Here's how the part is built. I have some questions about the finished solid (model axes, mm). A direction names the side the tool comes from. Coordinates: 2 decimals unless noted, no trailing zeros. Loops run counter-clockwise (first coordinate to the right, second up) from the corner with the lowest first, then second, coordinate; pieces in that order, holes last. Notation, with made-up numbers: (47, 73.25) - (81, 73.25) arc R19 ccw to (81, 88.25) - close; hole circle Ø7 at (-16.75, -38.75). An arc over 180 degrees is marked (long way). Use a Markdown table: item, result.
```python
from build123d import *

# Parameters (mm, degrees)
SKETCH1_W          = 50.8
SKETCH1_H          = 28.575
EXTRUDE1_DEPTH     = 65.8368
LPATTERN1_COUNT    = 2
LPATTERN1_PITCH    = 46.99
SKETCH5_R          = 13.5001
EXTRUDE2_DEPTH     = 5.969
SKETCH6_W          = 6.3373
SKETCH6_H          = 16.891
CUT_EXTRUDE4_DEPTH = 30.48
HOLE1_D            = 7.137
HOLE1_DEPTH        = 65.8368
HOLE2_D            = 7.137
HOLE2_DEPTH        = 28.575
EXTRUDE3_DEPTH     = 6.78


with BuildPart() as part:
    # Sketch1 → Extrude1 (new body)
    with BuildSketch(Plane(origin=(0, 0, 0), x_dir=(0, 0, -1), z_dir=(1, 0, 0))):
        with Locations((2.3876, 0)):
            Rectangle(SKETCH1_W, SKETCH1_H)
    extrude(amount=EXTRUDE1_DEPTH)

    # S2D0002 → Cut-Revolve1 (revolve, cut)
    with BuildSketch(Plane(origin=(0, 4.7625, 0), x_dir=(-1, 0, 0), z_dir=(0, 1, 0)), mode=Mode.PRIVATE) as cut_revolve1_sk:
        Polygon((-14.5415, -27.5336), (-18.161, -27.5336), (-18.161, -27.7876), (-9.525, -27.7876), (-9.525, -14.0716), (-13.9446, -14.0716), (-13.9446, -26.9113), (-14.5415, -27.5082), align=None)
    cut_revolve1 = revolve(cut_revolve1_sk.sketch.rotate(Axis((9.525, 4.7625, -19.13842003), (0, 0, 1)), 180), axis=Axis((9.525, 4.7625, -19.13842003), (0, 0, 1)), mode=Mode.SUBTRACT)  # turned: the seam where the file's is

    # LPattern1: Cut-Revolve1 ×2
    with Locations(*[(i * LPATTERN1_PITCH, 0, 0) for i in range(1, LPATTERN1_COUNT)]):
        add(cut_revolve1, mode=Mode.SUBTRACT)

    # Sketch5 → Extrude2 (add)
    with BuildSketch(Plane.ZY):
        Circle(SKETCH5_R)
    extrude(amount=EXTRUDE2_DEPTH)

    # Sketch6 → Revolve1 (revolve)
    with BuildSketch(Plane(origin=(0, 0, 0), x_dir=(0, 0, 1), z_dir=(0, -1, 0)), mode=Mode.PRIVATE) as revolve1_sk:
        with Locations((-3.16865, 14.4145)):
            Rectangle(SKETCH6_W, SKETCH6_H)
    revolve(revolve1_sk.sketch.rotate(Axis((5.754582971, 0, 0), (-1, 0, 0)), 180), axis=Axis((5.754582971, 0, 0), (-1, 0, 0)))  # turned: the seam where the file's is

    # S2D0001 → Cut-Revolve4 (revolve, cut)
    with BuildSketch(Plane(origin=(-18.511260017, 3.2639, 0), x_dir=(0, 1, 0), z_dir=(0, 0, 1)), mode=Mode.PRIVATE) as cut_revolve4_sk:
        Polygon((-0.7493, 2.984923177), (-0.7493, -11.653260017), (-3.2639, -13.16418413), (-3.2639, 4.348739983), (0.0381, 4.348739983), align=None)
    revolve(cut_revolve4_sk.sketch.rotate(Axis((0, 0, 0), (-1, 0, 0)), 90), axis=Axis((0, 0, 0), (-1, 0, 0)), mode=Mode.SUBTRACT)  # turned: the seam where the file's is

    # Sketch8 → Cut-Revolve5 (revolve, cut)
    with BuildSketch(Plane(origin=(0, 0, 0), x_dir=(0, 0, -1), z_dir=(0, 1, 0)), mode=Mode.PRIVATE) as cut_revolve5_sk:
        with BuildLine():
            Line((-6.3373, 16.5354), (-6.096, 17.2974))
            Line((-6.096, 17.2974), (-6.096, 21.844))
            ThreePointArc((-6.096, 21.844), (-5.995678675, 22.387796865), (-5.707922533, 22.86))
            Line((-5.707922533, 22.86), (-6.3373, 22.86))
            Line((-6.3373, 22.86), (-6.3373, 16.5354))
        make_face()
    revolve(cut_revolve5_sk.sketch.rotate(Axis((-12.65936, 0, 0), (-1, 0, 0)), 180), axis=Axis((-12.65936, 0, 0), (-1, 0, 0)), mode=Mode.SUBTRACT)  # turned: the seam where the file's is

    # Sketch12 → Cut-Extrude4 (cut, symmetric)
    with BuildSketch(Plane(origin=(0, 0, 0), x_dir=(0, -1, 0), z_dir=(0, 0, -1))):
        Polygon((5.461, 22.86), (5.461, 18.0848), (6.096, 17.4498), (6.096, 22.86), align=None)
        Polygon((-5.461, 22.86), (-5.461, 18.0848), (-6.096, 17.4498), (-6.096, 22.86), align=None)
    extrude(amount=CUT_EXTRUDE4_DEPTH, both=True, mode=Mode.SUBTRACT)

    # Hole1
    with Locations(Plane.ZY):
        with Locations((-16.6878, -7.9248), (16.6624, 7.9502)):
            Hole(HOLE1_D / 2, depth=HOLE1_DEPTH)

    # Hole2
    with Locations(Plane(origin=(0, 14.2875, 0), x_dir=(-1, 0, 0), z_dir=(0, 1, 0))):
        with Locations((-23.3172, -16.6878), (-23.3172, 16.6624)):
            Hole(HOLE2_D / 2, depth=HOLE2_DEPTH)

    # Sketch18 → Extrude3 (add)
    with BuildSketch(Plane(origin=(0, 0, -27.5336), x_dir=(-1, 0, 0), z_dir=(0, 0, -1))):
        Polygon((-2.54, 8.79529163), (-9.525, 12.828083261), (-16.51, 8.79529163), (-16.51, 0.72970837), (-9.525, -3.303083261), (-2.54, 0.72970837), align=None)
    extrude(amount=EXTRUDE3_DEPTH)

    # Sketch19 → Cut-Revolve6 (revolve, cut)
    with BuildSketch(Plane(origin=(0, 4.7625, 0), x_dir=(-1, 0, 0), z_dir=(0, 1, 0)), mode=Mode.PRIVATE) as cut_revolve6_sk:
        with BuildLine():
            Line((-15.748, -34.3136), (-15.748, -36.7266))
            Line((-15.748, -36.7266), (-18.923, -36.7266))
            Line((-18.923, -36.7266), (-18.923, -33.5516))
            Line((-18.923, -33.5516), (-16.51, -33.5516))
            ThreePointArc((-16.51, -33.5516), (-16.286815367, -34.090415367), (-15.748, -34.3136))
        make_face()
    revolve(cut_revolve6_sk.sketch.rotate(Axis((9.525, 4.7625, -18.51025594), (0, 0, -1)), 180), axis=Axis((9.525, 4.7625, -18.51025594), (0, 0, -1)), mode=Mode.SUBTRACT)  # turned: the seam where the file's is


solid = part.part
```
Q1. If we mould it in two halves opening along Z, with no side actions, what happens to faces 6 (the face through (56, 5, -14.072)), 7 (the face through (-21, 5.461, 0)), 8 (the face through (22.54, -11.86, -20.17)), 9 (the face through (-11.326, -6.187, -1.374))? For each: pulls with the +Z half, pulls with the -Z half, needs draft (parallel to the pull), parting line crosses it, or undercut.
Check values:
| item | result |
|---|---|
| face 6 | pulls with the -Z half |
| face 7 | needs draft |
| face 8 | undercut |
| face 9 | parting line crosses it |
Q2. I want a section at B-B, the plane z = -24. Write out the boundary of the cut face in (x, y) (1 decimal).
Check values:
| item | result |
|---|---|
| outline | (0, -14.3) - (65.8, -14.3) - (65.8, 14.3) - (0, 14.3) - close; hole circle Ø8.8 at (9.5, 4.8); hole circle Ø8.8 at (56.5, 4.8) |
Q3. I want a section at D-D, the plane x = 26. Write out the boundary of the cut face in (y, z), then the cut area to 3 significant figures.
Check values:
| item | result |
|---|---|
| outline | (-14.29, -27.79) - (14.29, -27.79) - (14.29, -19.04) - (-5.24, -19.04) arc R3.57 cw to (-10.61, -19.04) - (-14.29, -19.04) - close; (-14.29, -14.33) - (-10.61, -14.33) arc R3.57 cw to (-5.24, -14.33) - (14.29, -14.33) - (14.29, 14.31) - (10.63, 14.31) arc R3.57 cw to (5.27, 14.31) - (-14.29, 14.31) - close; (-14.29, 19.02) - (5.27, 19.02) arc R3.57 cw to (10.63, 19.02) - (14.29, 19.02) - (14.29, 23.01) - (-14.29, 23.01) - close |
| area | 1,160 mm^2 |
Q4. I want a section at A-A, the plane z = -15.5. Write out the boundary of the cut face in (x, y) (1 decimal), then the cut area to 3 significant figures.
Check values:
| item | result |
|---|---|
| outline | (0, -14.3) - (20, -14.3) - (20, -11.3) - (0, -11.3) - close; (0, -4.6) - (20, -4.6) - (20, 14.3) - (0, 14.3) - close; (26.7, -14.3) - (65.8, -14.3) - (65.8, -11.3) - (26.7, -11.3) - close; (26.7, -4.6) - (65.8, -4.6) - (65.8, 14.3) - (26.7, 14.3) - close; hole circle Ø8.8 at (9.5, 4.8); hole circle Ø8.8 at (56.5, 4.8) |
| area | 1,170 mm^2 |
Q5. Will these pins go through, and if not, where does the flat tip stop? P1, Ø8.5, axis at x = 22.5, y = -6.5, coming from the -Z side; P2, Ø6.5, axis at y = 7.95, z = 16.66, coming from the -X side; P3, Ø10, axis at x = -11, y = -2, coming from the +Z side; P4, Ø7, axis at x = 54.5, y = 4, coming from the -Z side.
Check values:
| item | result |
|---|---|
| P1 | z = -27.79 |
| P2 | through |
| P3 | z = 6.34 |
| P4 | z = -27.53 |
Q6. Please list where these lines run through material, in increasing order: L1, parallel to X at y = -11.75, z = -16.5; L2, parallel to Z at x = 40, y = -7.75; L3, parallel to Y at x = 42, z = 16.5 (1 decimal). Write a range as from..to.
Check values:
| item | result |
|---|---|
| L1 | 0..19.75, 26.88..65.84 |
| L2 | -27.79..-20.25, -13.12..23.01 |
| L3 | -14.3..4.4, 11.5..14.3 |
Q7. I want a section at C-C, the plane z = 15.5. Write out the boundary of the cut face in (x, y).
Check values:
| item | result |
|---|---|
| outline | (0, -14.29) - (19.94, -14.29) - (19.94, 4.58) - (0, 4.58) - close; (0, 11.32) - (19.94, 11.32) - (19.94, 14.29) - (0, 14.29) - close; (26.69, -14.29) - (65.84, -14.29) - (65.84, 4.58) - (26.69, 4.58) - close; (26.69, 11.32) - (65.84, 11.32) - (65.84, 14.29) - (26.69, 14.29) - close |
Q8. Which directions (+Z, -Z, +X, -X, +Y, -Y) give clear straight access to the entire face, cutting with the end or side of a thin tool? Please do faces 1 (the face through (44.875, -7.768, -13.123)), 2 (the face through (16, 8, -33.552)), 3 (the face through (60.93, 4.57, -20.58)), 4 (the face through (9, 5, -14.072)), 5 (the face through (9.5, -2.4, -33.552)).
Check values:
| item | result |
|---|---|
| face 1 | +X, -X |
| face 2 | -Z, +X, +Y |
| face 3 | -Z |
| face 4 | none |
| face 5 | -Z, -Y |
